from build123d import *

# Parameters (mm, degrees)
BOSS_EXTRUDE1_DEPTH         = 40
CUT_EXTRUDE2_REACH          = 50.564
M6_TAPPED_HOLE1_D           = 5
M6_TAPPED_HOLE1_DEPTH       = 17
M6_TAPPED_HOLE1_CSINK_D     = 6.05
M6_TAPPED_HOLE1_CSINK_ANGLE = 90
M6_TAPPED_HOLE1_TIP         = 1.502151548


with BuildPart() as part:
    # Sketch1 → Boss-Extrude1 (new body)
    with BuildSketch(Plane(origin=(0, 0, 0), x_dir=(1, 0, 0), z_dir=(0, 1, 0))):
        with BuildLine():
            Line((-5.5, -26.5), (5.5, -26.5))
            ThreePointArc((5.5, -26.5), (6.914213562, -25.914213562), (7.5, -24.5))
            Line((7.5, -24.5), (7.5, 24.5))
            ThreePointArc((7.5, 24.5), (6.914213562, 25.914213562), (5.5, 26.5))
            Line((5.5, 26.5), (-5.5, 26.5))
            ThreePointArc((-5.5, 26.5), (-6.914213562, 25.914213562), (-7.5, 24.5))
            Line((-7.5, 24.5), (-7.5, -24.5))
            ThreePointArc((-7.5, -24.5), (-6.914213562, -25.914213562), (-5.5, -26.5))
        make_face()
    extrude(amount=-BOSS_EXTRUDE1_DEPTH)

    # Sketch5 → Cut-Extrude2 (cut, up to next)
    with BuildSketch(Plane(origin=(0, 0, 0), x_dir=(1, 0, 0), z_dir=(0, 1, 0)), mode=Mode.PRIVATE) as cut_extrude2_sk1:
        with BuildLine():
            Line((-2.55, -12.05), (-2.55, 12.05))
            ThreePointArc((-2.55, 12.05), (0, 14.6), (2.55, 12.05))
            Line((2.55, 12.05), (2.55, -12.05))
            ThreePointArc((2.55, -12.05), (0, -14.6), (-2.55, -12.05))
        make_face()
    cut_extrude2_tool1 = extrude(cut_extrude2_sk1.sketch, amount=-CUT_EXTRUDE2_REACH, mode=Mode.PRIVATE) & part.part
    add(cut_extrude2_tool1.solids().sort_by_distance((0, 0, 0))[0], mode=Mode.SUBTRACT)

    # Cut-Sweep1: sweep along a path in Sketch8
    with BuildLine(Plane(origin=(0, 0, 0), x_dir=(1, 0, 0), z_dir=(0, 1, 0))) as cut_sweep1_path:
        Line((-2.55, 12.05), (-2.55, -12.05))
        ThreePointArc((-2.55, -12.05), (0, -14.6), (2.55, -12.05))
        Line((2.55, -12.05), (2.55, 12.05))
        ThreePointArc((2.55, 12.05), (0, 14.6), (-2.55, 12.05))
    # Sketch7 → Cut-Sweep1 (sweep, cut)
    with BuildSketch(Plane.XY):
        Polygon((2.55, -3.2), (3.192346389, -40), (2.55, -40), align=None)
    sweep(path=cut_sweep1_path.line, mode=Mode.SUBTRACT)

    # M6 Tapped Hole1
    with Locations(Plane(origin=(0, -40, 0), x_dir=(-1, 0, 0), z_dir=(0, -1, 0))):
        with Locations((0, 22.5), (0, -22.5)):
            CounterSinkHole(M6_TAPPED_HOLE1_D / 2, M6_TAPPED_HOLE1_CSINK_D / 2, depth=M6_TAPPED_HOLE1_DEPTH, counter_sink_angle=M6_TAPPED_HOLE1_CSINK_ANGLE)
            with Locations((0, 0, -(M6_TAPPED_HOLE1_DEPTH + M6_TAPPED_HOLE1_TIP / 2))):  # 118° drill point
                Cone(0, M6_TAPPED_HOLE1_D / 2, M6_TAPPED_HOLE1_TIP, mode=Mode.SUBTRACT)


solid = part.part
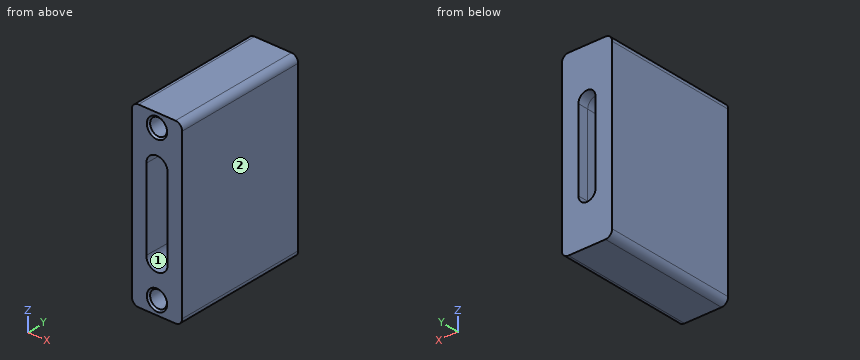
Read the model definition and answer for the solid it produces. Units are mm, in the model's axes. Face numbers are marked on the shaded views. A direction names the side the tool comes from. Coordinates: 2 decimals unless noted, no trailing zeros. Loops run counter-clockwise (first coordinate to the right, second up) from the corner with the lowest first, then second, coordinate; pieces in that order, holes last. Notation, with made-up numbers: (85, 26) -> (122, 26) arc R16 cw to (122, 50) -> close; hole circle Ø2 at (14, 29.25). An arc over 180 degrees is marked (long way). Answer in a Markdown table with one row per item.
Item 1: A cutting plane is placed at B-B on y = -36. Determine the outline of the cut face in (x, z).
Returned:
| item | result |
|---|---|
| outline | (-7.5, -24.5) arc R2 ccw to (-5.5, -26.5) -> (5.5, -26.5) arc R2 ccw to (7.5, -24.5) -> (7.5, 24.5) arc R2 ccw to (5.5, 26.5) -> (-5.5, 26.5) arc R2 ccw to (-7.5, 24.5) -> close; hole (-3.12, -12.05) arc R3.12 ccw to (3.12, -12.05) -> (3.12, 12.05) arc R3.12 ccw to (-3.12, 12.05) -> close; hole circle Ø5 at (0, -22.5); hole circle Ø5 at (0, 22.5) |
Item 2: A cutting plane is placed at A-A on y = -11. Determine the outline of the cut face in (x, z).
Returned:
| item | result |
|---|---|
| outline | (-7.5, -24.5) arc R2 ccw to (-5.5, -26.5) -> (5.5, -26.5) arc R2 ccw to (7.5, -24.5) -> (7.5, 24.5) arc R2 ccw to (5.5, 26.5) -> (-5.5, 26.5) arc R2 ccw to (-7.5, 24.5) -> close; hole (-2.69, -12.05) arc R2.69 ccw to (2.69, -12.05) -> (2.69, 12.05) arc R2.69 ccw to (-2.69, 12.05) -> close |
Item 3: For the marked faces 1 and 2, determine the directions among +Z, -Z, +X, -X, +Y, -Y from which every point of the face is accessible in a straight line to the end or side of a thin tool.
Returned:
| item | result |
|---|---|
| face 1 | -Y |
| face 2 | +Z, -Z, +X, +Y, -Y |
Item 4: A cutting plane is placed at C-C on y = -31.5. Determine the outline of the cut face in (x, z), plus the area to 3 significant figures.
Returned:
| item | result |
|---|---|
| outline | (-7.5, -24.5) arc R2 ccw to (-5.5, -26.5) -> (5.5, -26.5) arc R2 ccw to (7.5, -24.5) -> (7.5, 24.5) arc R2 ccw to (5.5, 26.5) -> (-5.5, 26.5) arc R2 ccw to (-7.5, 24.5) -> close; hole (-3.04, -12.05) arc R3.04 ccw to (3.04, -12.05) -> (3.04, 12.05) arc R3.04 ccw to (-3.04, 12.05) -> close; hole circle Ø5 at (0, -22.5); hole circle Ø5 at (0, 22.5) |
| area | 576 mm^2 |
Item 5: Straight lines are drawn through the part: line 1 along X through (y, z) = (-30.25, -22.5); line 2 along X through (y, z) = (-3, 4.5); line 3 along Z through (x, y) = (0, -33). For each, find the intervals that lie inside material, in ascending order. Write a range as [from, to].
Returned:
| item | result |
|---|---|
| line 1 | x = [-7.5, -2.5], [2.5, 7.5] |
| line 2 | x = [-7.5, -2.55], [2.55, 7.5] |
| line 3 | z = [-26.5, -25], [-20, -15.12], [15.12, 20], [25, 26.5] |
